```python
from build123d import *

# Parameters (mm, degrees)
ESBO_O1_R                = 1.6
RESSALTO_EXTRUS_O1_DEPTH = 3


with BuildPart() as part:
    # Esboço1 → Ressalto-extrusão1 (new body)
    with BuildSketch(Plane.XZ.offset(6)):
        Polygon((17.1, 41.9), (7.5, 41.9), (7.5, 47.9), (-7.5, 47.9), (-7.5, 41.9), (-17.1, 41.9), (-17.1, -3.6), (-7.5, -3.6), (-7.5, -9.6), (7.5, -9.6), (7.5, -3.6), (17.1, -3.6), align=None)
        with Locations((-12.5, 20.9)):
            Circle(ESBO_O1_R, mode=Mode.SUBTRACT)
        Circle(ESBO_O1_R, mode=Mode.SUBTRACT)
        with Locations((12.5, 20.9)):
            Circle(ESBO_O1_R, mode=Mode.SUBTRACT)
    extrude(amount=-RESSALTO_EXTRUS_O1_DEPTH)


solid = part.part
```
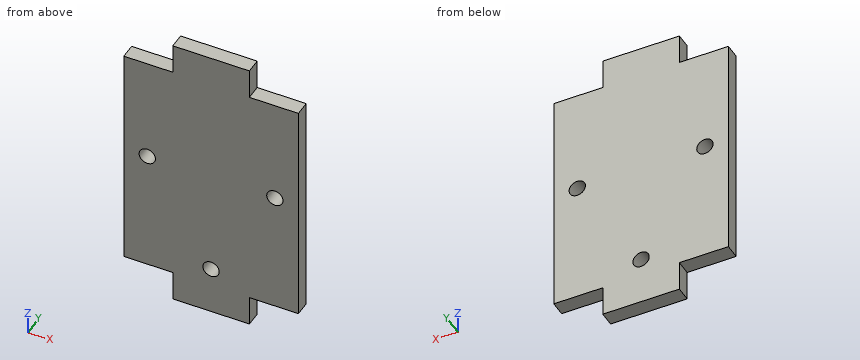
The listing builds one solid part. Answer for the finished solid, in the listing's coordinates (mm). Coordinates: 2 decimals unless noted, no trailing zeros. Write each loop counter-clockwise with the first axis right and the second up, starting at its lowest first coordinate (ties: lowest second). Pieces come first, ordered by that corner, then holes. Notation, with made-up numbers: (33.5, 83.25) - (65.5, 83.25) arc R18 ccw to (65.5, 90.25) - close; hole circle Ø6 at (17.25, 68). An arc over 180 degrees is marked (long way). Return JSON: item names as keys, results as strings. Group by question number.
1. A cutting plane is placed at C-C, the plane z = 0. Determine the outline of the cut face in (x, y).
2. A cutting plane is placed at A-A, the plane x = 0. Determine the outline of the cut face in (y, z).
3. A cutting plane is placed at D-D, the plane y = -4.15. Determine the outline of the cut face in (x, z).
4. Given pin 1 (1.5 mm diameter, centred on y = -4.5, z = -5.5, fed in from +X); pin 2 (3 mm diameter, centred on x = 0, z = 0, fed in from +Y); pin 3 (1.5 mm diameter, centred on x = 11.5, y = -5, fed in from -Z); pin 4 (1.5 mm diameter, centred on x = -11.5, y = -4.5, fed in from +Z), each flat-ended and moving along its own axis, determine where each tip first touches the part or whether it passes through.
5. Straight lines are drawn through the part: L1, parallel to Z at x = 12.5, y = -4.85; L2, parallel to X at y = -4.25, z = 20.5; L3, parallel to Z at x = 0, y = -4.45. For each, find the intervals that lie inside material, in ascending order.
6. A cutting plane is placed at B-B, the plane z = 20.9. Determine the outline of the cut face in (x, y), plus the area to 3 significant figures.
Ans:
{
 "1": {"outline": "(-17.1, -6) - (-1.6, -6) - (-1.6, -3) - (-17.1, -3) - close; (1.6, -6) - (17.1, -6) - (17.1, -3) - (1.6, -3) - close"},
 "2": {"outline": "(-6, -9.6) - (-3, -9.6) - (-3, -1.6) - (-6, -1.6) - close; (-6, 1.6) - (-3, 1.6) - (-3, 47.9) - (-6, 47.9) - close"},
 "3": {"outline": "(-17.1, -3.6) - (-7.5, -3.6) - (-7.5, -9.6) - (7.5, -9.6) - (7.5, -3.6) - (17.1, -3.6) - (17.1, 41.9) - (7.5, 41.9) - (7.5, 47.9) - (-7.5, 47.9) - (-7.5, 41.9) - (-17.1, 41.9) - close; hole circle Ø3.2 at (-12.5, 20.9); hole circle Ø3.2 at (0, 0); hole circle Ø3.2 at (12.5, 20.9)"},
 "4": {"pin 1": "x = 7.5", "pin 2": "through", "pin 3": "z = -3.6", "pin 4": "z = 41.9"},
 "5": {"L1": "-3.6 to 19.3, 22.5 to 41.9", "L2": "-17.1 to -14.05, -10.95 to 10.95, 14.05 to 17.1", "L3": "-9.6 to -1.6, 1.6 to 47.9"},
 "6": {"outline": "(-17.1, -6) - (-14.1, -6) - (-14.1, -3) - (-17.1, -3) - close; (-10.9, -6) - (10.9, -6) - (10.9, -3) - (-10.9, -3) - close; (14.1, -6) - (17.1, -6) - (17.1, -3) - (14.1, -3) - close", "area": "83.4 mm²"}
}
